from build123d import *

# Parameters (mm, degrees)
SKETCH1_R           = 14.2875
BOSS_EXTRUDE1_DEPTH = 6.35
SKETCH2_R           = 15.8877
BOSS_EXTRUDE2_DEPTH = 1.5748


with BuildPart() as part:
    # Sketch1 → Boss-Extrude1 (new body)
    with BuildSketch(Plane(origin=(0, 0, 0), x_dir=(1, 0, 0), z_dir=(0, 1, 0))):
        Circle(SKETCH1_R)
        Polygon((7.332348419, 0), (3.666174209, 6.35), (-3.666174209, 6.35), (-7.332348419, 0), (-3.666174209, -6.35), (3.666174209, -6.35), align=None, mode=Mode.SUBTRACT)
    extrude(amount=BOSS_EXTRUDE1_DEPTH)

    # Sketch2 → Boss-Extrude2 (add)
    with BuildSketch(Plane.XZ):
        Circle(SKETCH2_R)
        Polygon((-7.332348419, 0), (-3.666174209, -6.35), (3.666174209, -6.35), (7.332348419, 0), (3.666174209, 6.35), (-3.666174209, 6.35), align=None, mode=Mode.SUBTRACT)
    extrude(amount=BOSS_EXTRUDE2_DEPTH)


solid = part.part
For this review, take the finished solid that the model builds, in its own axes (mm). A direction names the side the tool comes from. Round coordinates to 2 decimals unless told otherwise and drop trailing zeros. Write each loop counter-clockwise with the first axis right and the second up, starting at its lowest first coordinate (ties: lowest second). Pieces come first, ordered by that corner, then holes. Notation, with made-up numbers: (-16, 78) - (31, 78) arc R20 cw to (31, 87) - close; hole circle Ø10 at (0, -15). An arc over 180 degrees is marked (long way). Write item = value, one per line. Start each with the question number.
1. Consider section B-B on y = -1. State the section outline as (x, z) points.
2. Consider section C-C on z = -4.5. State the section outline as (x, y) points, plus the area to 3 significant figures.
3. Consider section A-A on x = 0. State the section outline as (y, z) points.
4. Wall thickness on L1, parallel to Z at x = 5.5, y = 1.75; L2, parallel to X at y = 4, z = 5.5; L3, parallel to X at y = 0.75, z = -6: over which ranges is each line inside the solid? List them lowest first.
5. For faces 1 (the face through (-14.274, 3.131, -0.628)), 2 (the face through (0, 2, 6.35)), 3 (the face through (0, -1.575, -7)), list the 3-axis set-ups (+Z, -Z, +X, -X, +Y, -Y) from which the entire face can be reached by the end or side of a thin tool; tool diameter is ignored.
6. For pin 1 Ø4 at (y, z) = (4, -2) entering from -X; pin 2 Ø3 at (y, z) = (4.5, 4.5) entering from +X, all flat-tipped, find the tip position at first contact; note any pin that passes through.
7. Draft analysis for pull direction Z (two halves, no side actions). For faces 4 (the face through (-3.44, -0.78, -15.51)), 5 (the face through (5.525, 2.443, 3.131)), 6 (the face through (-11.84, 0, 8.31)), state which applies: released by +Z, released by -Z, zero draft, split by the parting line, or undercut.
Evaluation:
q1.outline = circle Ø31.78 at (0, 0); hole (-7.33, 0) - (-3.67, -6.35) - (3.67, -6.35) - (7.33, 0) - (3.67, 6.35) - (-3.67, 6.35) - close
q2.outline = (-15.24, -1.57) - (-4.73, -1.57) - (-4.73, 6.35) - (-13.56, 6.35) - (-13.56, 0) - (-15.24, 0) - close; (4.73, -1.57) - (15.24, -1.57) - (15.24, 0) - (13.56, 0) - (13.56, 6.35) - (4.73, 6.35) - close
q2.area = 145 mm2
q3.outline = (-1.57, -15.89) - (0, -15.89) - (0, -14.29) - (6.35, -14.29) - (6.35, -6.35) - (-1.57, -6.35) - close; (-1.57, 6.35) - (6.35, 6.35) - (6.35, 14.29) - (0, 14.29) - (0, 15.89) - (-1.57, 15.89) - close
q4.L1 = -13.19 to -3.17, 3.17 to 13.19
q4.L2 = -13.19 to -4.16, 4.16 to 13.19
q4.L3 = -12.97 to -3.87, 3.87 to 12.97
q5.face_1 = +Y
q5.face_2 = +Y, -Y
q5.face_3 = +Z, -Z, +X, -X, -Y
q6.pin_1 = -14.29
q6.pin_2 = 13.97
q7.face_4 = split by the parting line
q7.face_5 = undercut
q7.face_6 = zero draft
